```python
from build123d import *

# Parameters (mm, degrees)
SKETCH1_W           = 100
SKETCH1_H           = 100
BOSS_EXTRUDE1_DEPTH = 50
SKETCH2_W           = 8.5
SKETCH2_H           = 113.5
BOSS_EXTRUDE2_DEPTH = 8.5
FILLET1_R           = 1


with BuildPart() as part:
    # Sketch1 → Boss-Extrude1 (new, symmetric)
    with BuildSketch(Plane(origin=(0, 0, 0), x_dir=(1, 0, 0), z_dir=(0, 1, 0))):
        Rectangle(SKETCH1_W, SKETCH1_H)
    extrude(amount=BOSS_EXTRUDE1_DEPTH, both=True)

    # Sketch2 → Boss-Extrude2 (add)
    with BuildSketch(Plane(origin=(0, 0, 50), x_dir=(1, 0, 0), z_dir=(0, 0, -1))):
        with Locations((-45.75, 0.25)):
            Rectangle(SKETCH2_W, SKETCH2_H)
        with Locations((45.75, 0.25)):
            Rectangle(SKETCH2_W, SKETCH2_H)
    boss_extrude2 = extrude(amount=BOSS_EXTRUDE2_DEPTH)

    # Mirror1: Boss-Extrude2 across plane
    add(boss_extrude2.mirror(Plane.XY))

    # Fillet1
    fillet1_edges = [part.edges().sort_by_distance(p)[0] for p in [
        (50, -0.25, 50),
        (-50, -0.25, 50),
        (-50, -0.25, -50),
        (50, -0.25, -50),
    ]]
    fillet(fillet1_edges, radius=FILLET1_R)


solid = part.part
```
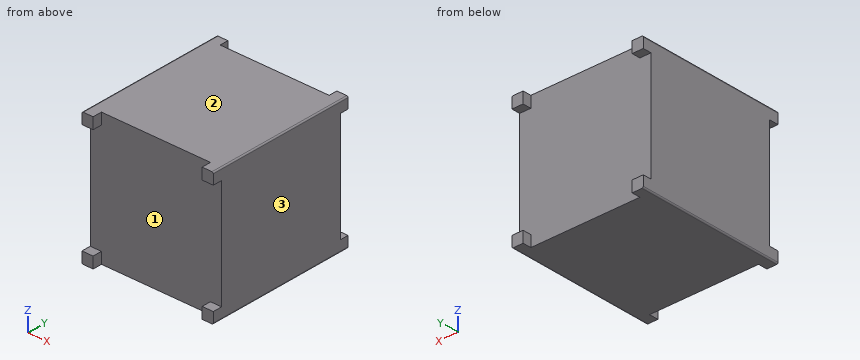
The model under review builds one solid part; all positions refer to its coordinate system, in mm. Face numbers are marked on the shaded views. Round coordinates to 2 decimals unless told otherwise and drop trailing zeros. Loops run counter-clockwise (first coordinate to the right, second up) from the corner with the lowest first, then second, coordinate; pieces in that order, holes last. Notation, with made-up numbers: (66, 80) -> (114, 80) arc R13 cw to (114, 103) -> close; hole circle Ø4 at (71, -33). An arc over 180 degrees is marked (long way). Answer as a JSON object with one key per item and string values. Group by question number.
1) For line 1 (Y direction, x = -45, z = 29), list the stretches that pass through material, from the lowest coordinate up. Write a range as [from, to].
2) We need section A-A on x = 43.5. Write out the cut boundary in (y, z), then the cut area to 3 significant figures.
3) We need section B-B on z = 38.5. Write out the cut boundary in (x, y), then the cut area to 3 significant figures.
4) For pin 1 Ø1 at (x, z) = (10.5, -29) entering from -Y; pin 2 Ø10 at (x, z) = (14.5, -3.5) entering from +Y, all flat-tipped, find the tip position at first contact; note any pin that passes through.
5) Mouldability with a two-part tool opening along Z and no side actions: class the marked faces 1, 2 and 3 as released by +Z, released by -Z, zero draft, split by the parting line, or undercut.
Result set:
{
 "1": {"line 1": "[-50, 50]"},
 "2": {"outline": "(-57, -50) -> (56.5, -50) -> (56.5, -41.5) -> (50, -41.5) -> (50, 41.5) -> (56.5, 41.5) -> (56.5, 50) -> (-57, 50) -> (-57, 41.5) -> (-50, 41.5) -> (-50, -41.5) -> (-57, -41.5) -> close", "area": "10,200 mm²"},
 "3": {"outline": "(-50, -50) -> (50, -50) -> (50, 50) -> (-50, 50) -> close", "area": "10,000 mm²"},
 "4": {"pin 1": "y = -50", "pin 2": "y = 50"},
 "5": {"face 1": "undercut", "face 2": "released by +Z", "face 3": "zero draft"}
}
